Autodesk Inventor part; units mm, degrees
ref_plane "a10_to_bolt_XY" through (0, 9, 75) normal (0, 1, 0) x (1, 0, 0)
ref_plane "a10_to_bolt_YZ" through (0, 9, 75) normal (1, 0, 0) x (0, 0, -1)
ref_plane "a10_to_bolt_ZX" through (0, 9, 75) normal (0, 0, -1) x (0, 1, 0)
sketch "Sketch_1" plane through (0, 0, 0) normal (1, 0, 0) x (0, 1, 0)
  line L0 (0, 55) -> (0, 0)
  line L1 (0, 0) -> (85, 0)
  line L2 (85, 0) -> (85, 9)
  line L3 (85, 9) -> (33, 9)
  line L4 (33, 9) -> (9, 33)
  line L5 (9, 33) -> (9, 55)
  line L6 (9, 55) -> (0, 55)
  arc A0 (8.7071, 30.4645) -> (7, 29.7574) centre (8, 29.7574) ccw
  line L7 (7, 29.7574) -> (7, 12)
  line L8 (7, 12) -> (8.9, 12)
  arc A1 (12.5383, 15.0529) -> (8.9, 12) centre (12, 12) ccw
  line L9 (12.5383, 15.0529) -> (12.3647, 14.0681)
  arc A2 (12.3647, 14.0681) -> (14.0681, 12.3647) centre (12.5843, 12.5843) ccw
  line L10 (14.0681, 12.3647) -> (15.0529, 12.5383)
  arc A3 (12, 8.9) -> (15.0529, 12.5383) centre (12, 12) ccw
  line L11 (12, 8.9) -> (12, 7)
  line L12 (12, 7) -> (29.7574, 7)
  arc A4 (29.7574, 7) -> (30.4645, 8.7071) centre (29.7574, 8) ccw
  line L13 (30.4645, 8.7071) -> (8.7071, 30.4645)
extrude "Extrusion1" add sketch "Sketch_1" along normal mid plane 20
sketch "Sketch_10" plane through (0, 12, 0) normal (0, 1, 0) x (1, 0, 0)
  line L0 (-10, -12) -> (10, -12)
  line L1 (10, -12) -> (10, -14.5)
  line L2 (10, -14.5) -> (9.567, -14.067)
  line L3 (9.567, -14.067) -> (-9.567, -14.067)
  line L4 (-9.567, -14.067) -> (-10, -14.5)
  line L5 (-10, -14.5) -> (-10, -12)
  line L6 (-10, -12) -> (10, -12)
revolve "Revolution1" cut sketch "Sketch_10" angle 360 about axis through (-10, 12, 12) along (-1, 0, 0)
thread "Thread1"
sketch "Sketch3" plane through (10, 0, 0) normal (0, 0, -1) x (-1, 0, 0)
  point P0 (10, 45)
hole "Hole1" at (0, 45, 0) direction (0, 0, 1) diameter 7 depth 9
sketch "Sketch4" plane through (-10, 0, 55) normal (0, -1, 0) x (1, 0, 0)
  point P0 (10, -10)
hole "Hole2" at (0, 0, 45) direction (0, 1, 0) diameter 7 depth 9
sketch "Sketch5" plane through (10, 0, 0) normal (0, 0, -1) x (-1, 0, 0)
  point P0 (10, 75)
hole "Hole3" at (0, 75, 0) direction (0, 0, 1) diameter 7 depth 9
ref_plane "a10_to_bolt_XY" through (0, 9, 75) normal (0, 1, 0) x (1, 0, 0)
ref_plane "a10_to_bolt_YZ" through (0, 9, 75) normal (1, 0, 0) x (0, 0, -1)
ref_plane "a10_to_bolt_ZX" through (0, 9, 75) normal (0, 0, -1) x (0, 1, 0)
ref_plane "a11_to_bolt_XY" through (0, 75, 9) normal (0, 0, 1) x (1, 0, 0)
ref_plane "a11_to_bolt_YZ" through (0, 75, 9) normal (1, 0, 0) x (0, 1, 0)
ref_plane "a11_to_bolt_ZX" through (0, 75, 9) normal (0, 1, 0) x (0, 0, 1)
ref_plane "a13_to_bolt_XY" through (20, 75, 9) normal (0, 0, 1) x (1, 0, 0)
ref_plane "a13_to_bolt_YZ" through (20, 75, 9) normal (1, 0, 0) x (0, 1, 0)
ref_plane "a13_to_bolt_ZX" through (20, 75, 9) normal (0, 1, 0) x (0, 0, 1)
ref_plane "a14_to_bolt_XY" through (-20, 75, 9) normal (0, 0, 1) x (1, 0, 0)
ref_plane "a14_to_bolt_YZ" through (-20, 75, 9) normal (1, 0, 0) x (0, 1, 0)
ref_plane "a14_to_bolt_ZX" through (-20, 75, 9) normal (0, 1, 0) x (0, 0, 1)
ref_plane "a15_to_bolt_XY" through (20, 45, 9) normal (0, 0, 1) x (1, 0, 0)
ref_plane "a15_to_bolt_YZ" through (20, 45, 9) normal (1, 0, 0) x (0, 1, 0)
ref_plane "a15_to_bolt_ZX" through (20, 45, 9) normal (0, 1, 0) x (0, 0, 1)
ref_plane "a16_to_bolt_XY" through (-20, 45, 9) normal (0, 0, 1) x (1, 0, 0)
ref_plane "a16_to_bolt_YZ" through (-20, 45, 9) normal (1, 0, 0) x (0, 1, 0)
ref_plane "a16_to_bolt_ZX" through (-20, 45, 9) normal (0, 1, 0) x (0, 0, 1)
ref_plane "a17_to_bolt_XY" through (20, 9, 75) normal (0, 1, 0) x (1, 0, 0)
ref_plane "a17_to_bolt_YZ" through (20, 9, 75) normal (1, 0, 0) x (0, 0, -1)
ref_plane "a17_to_bolt_ZX" through (20, 9, 75) normal (0, 0, -1) x (0, 1, 0)
ref_plane "a18_XY" through (-20, 9, 75) normal (0, 1, 0) x (1, 0, 0)
ref_plane "a18_YZ" through (-20, 9, 75) normal (1, 0, 0) x (0, 0, -1)
ref_plane "a18_ZX" through (-20, 9, 75) normal (0, 0, -1) x (0, 1, 0)
ref_plane "a19_to_bolt_XY" through (20, 9, 45) normal (0, 1, 0) x (1, 0, 0)
ref_plane "a19_to_bolt_YZ" through (20, 9, 45) normal (1, 0, 0) x (0, 0, -1)
ref_plane "a19_to_bolt_ZX" through (20, 9, 45) normal (0, 0, -1) x (0, 1, 0)
ref_plane "a1_to_bolt_XY" through (0, 45, 9) normal (0, 0, 1) x (1, 0, 0)
ref_plane "a1_to_bolt_YZ" through (0, 45, 9) normal (1, 0, 0) x (0, 1, 0)
ref_plane "a1_to_bolt_ZX" through (0, 45, 9) normal (0, 1, 0) x (0, 0, 1)
ref_plane "a20_to_bolt_XY" through (-20, 9, 45) normal (0, 1, 0) x (1, 0, 0)
ref_plane "a20_to_bolt_YZ" through (-20, 9, 45) normal (1, 0, 0) x (0, 0, -1)
ref_plane "a20_to_bolt_ZX" through (-20, 9, 45) normal (0, 0, -1) x (0, 1, 0)
ref_plane "a2_to_bolt_XY" through (0, 9, 45) normal (0, 1, 0) x (1, 0, 0)
ref_plane "a2_to_bolt_YZ" through (0, 9, 45) normal (1, 0, 0) x (0, 0, -1)
ref_plane "a2_to_bolt_ZX" through (0, 9, 45) normal (0, 0, -1) x (0, 1, 0)
ref_plane "a3_to_bolt_XY" through (0, 75, 9) normal (0, 0, 1) x (1, 0, 0)
ref_plane "a3_to_bolt_YZ" through (0, 75, 9) normal (1, 0, 0) x (0, 1, 0)
ref_plane "a3_to_bolt_ZX" through (0, 75, 9) normal (0, 1, 0) x (0, 0, 1)
ref_plane "a4_to_bolt_XY" through (0, 75, 9) normal (0, 0, 1) x (1, 0, 0)
ref_plane "a4_to_bolt_YZ" through (0, 75, 9) normal (1, 0, 0) x (0, 1, 0)
ref_plane "a4_to_bolt_ZX" through (0, 75, 9) normal (0, 1, 0) x (0, 0, 1)
ref_plane "a5_to_bolt_XY" through (0, 9, 75) normal (0, 1, 0) x (1, 0, 0)
ref_plane "a5_to_bolt_YZ" through (0, 9, 75) normal (1, 0, 0) x (0, 0, -1)
ref_plane "a5_to_bolt_ZX" through (0, 9, 75) normal (0, 0, -1) x (0, 1, 0)
ref_plane "a6_to_bolt_XY" through (0, 9, 75) normal (0, 1, 0) x (1, 0, 0)
ref_plane "a6_to_bolt_YZ" through (0, 9, 75) normal (1, 0, 0) x (0, 0, -1)
ref_plane "a6_to_bolt_ZX" through (0, 9, 75) normal (0, 0, -1) x (0, 1, 0)
ref_plane "a7_to_bolt_XY" through (0, 75, 9) normal (0, 0, 1) x (1, 0, 0)
ref_plane "a7_to_bolt_YZ" through (0, 75, 9) normal (1, 0, 0) x (0, 1, 0)
ref_plane "a7_to_bolt_ZX" through (0, 75, 9) normal (0, 1, 0) x (0, 0, 1)
ref_plane "a8_to_bolt_XY" through (0, 75, 9) normal (0, 0, 1) x (1, 0, 0)
ref_plane "a8_to_bolt_YZ" through (0, 75, 9) normal (1, 0, 0) x (0, 1, 0)
ref_plane "a8_to_bolt_ZX" through (0, 75, 9) normal (0, 1, 0) x (0, 0, 1)
ref_plane "a9_to_bolt_XY" through (0, 9, 75) normal (0, 1, 0) x (1, 0, 0)
ref_plane "a9_to_bolt_YZ" through (0, 9, 75) normal (1, 0, 0) x (0, 0, -1)
ref_plane "a9_to_bolt_ZX" through (0, 9, 75) normal (0, 0, -1) x (0, 1, 0)
ref_plane "bracket_to_dummy_XY" through (0, 0, 0) normal (0, 1, 0) x (1, 0, 0)
ref_plane "bracket_to_dummy_YZ" through (0, 0, 0) normal (1, 0, 0) x (0, 0, -1)
ref_plane "bracket_to_dummy_ZX" through (0, 0, 0) normal (0, 0, -1) x (0, 1, 0)
ref_plane "h12_to_bolt_XY" through (0, 9, 75) normal (0, 1, 0) x (1, 0, 0)
ref_plane "h12_to_bolt_YZ" through (0, 9, 75) normal (1, 0, 0) x (0, 0, -1)
ref_plane "h12_to_bolt_ZX" through (0, 9, 75) normal (0, 0, -1) x (0, 1, 0)
properties part number "HBLTF6-C_"
Source: CAD feature listing. Evaluate the final solid. Frame: model axes, mm. A direction names the side the tool comes from. Round coordinates to 2 decimals unless told otherwise and drop trailing zeros. Loops run counter-clockwise (first coordinate to the right, second up) from the corner with the lowest first, then second, coordinate; pieces in that order, holes last. Notation, with made-up numbers: M 84.5,25 L 127.5,25 A20 ccw 127.5,61 Z; hole C -29,22.25 d5. An arc over 180 degrees is marked long. Use a Markdown table: item, result. Add a question column.
1. Section query B-B on z = 45. Return the cut outline in (x, y), then the cut area to 3 significant figures.
2. Section query A-A on x = 0. Give the number of separate pieces and of enclosed holes in the cut face, then the cut area to 3 significant figures.
3. Contact query for flat-ended pins moving along their axis: P1, Ø8, axis at x = -1, y = 31, coming from the +Z side; P2, Ø3, axis at x = -4.5, y = 22.5, coming from the +Z side; P3, Ø6, axis at x = -3.5, z = 42.5, coming from the +Y side. Output: stop coordinate, or through.
4. Section query D-D on x = 8.5. Return the cut outline in (y, z), then the cut area to 3 significant figures.
5. Mould query, pull axis X, two halves, no side actions, for faces 1 (the flat face through (0, 85, 4)), 2 (the cylindrical face through (1.341, 78.233, 4.563)), 3 (the conical face through (-9.69, 10.507, 10.397)). Classes: pulls with the +X half, pulls with the -X half, needs draft (parallel to the pull), parting line crosses it, or undercut.
6. Reachability of faces 4 (the flat face through (0, 7, 21)), 5 (the conical face through (9.69, 10.397, 10.507)), 6 (the flat face through (0, 9, 41)) from +Z, -Z, +X, -X, +Y, -Y: full face, straight path, thin tool, end or side. Return the list, or none.
7. Line query: line 1 (Y direction, x = 0, z = 4.25); line 2 (X direction, y = 75, z = 2.5); line 3 (Y direction, x = -7.5, z = 11). Output: solid intervals per line, ascending.
Reported:
| question | item | result |
|---|---|---|
| 1 | outline | M -10,0 L -3.5,0 L -3.5,9 L -10,9 Z; M 3.5,0 L 10,0 L 10,9 L 3.5,9 Z |
| 1 | area | 117 mm² |
| 2 | separate pieces | 4 |
| 2 | enclosed holes | 1 |
| 2 | area | 995 mm² |
| 3 | P1 | stops at z = 15 |
| 3 | P2 | stops at z = 21 |
| 3 | P3 | stops at y = 9 |
| 4 | outline | M 0,0 L 85,0 L 85,9 L 33,9 L 9,33 L 9,55 L 0,55 Z; hole M 7,12 L 8.9,12 A3.1 cw 12.54,15.05 L 12.36,14.07 A1.5 ccw 12.27,14.05 A2.07 ccw long 14.05,12.27 A1.5 ccw 14.07,12.36 L 15.05,12.54 A3.1 cw 12,8.9 L 12,7 L 29.76,7 A1 ccw 30.46,8.71 L 8.71,30.46 A1 ccw 7,29.76 Z |
| 4 | area | 1,180 mm² |
| 5 | face 1 | needs draft |
| 5 | face 2 | undercut |
| 5 | face 3 | pulls with the -X half |
| 6 | face 4 | +X, -X |
| 6 | face 5 | +X |
| 6 | face 6 | +Z, +X, -X, +Y |
| 7 | line 1 | y = 0 to 41.5, 48.5 to 71.5, 78.5 to 85 |
| 7 | line 2 | x = -10 to -3.5, 3.5 to 10 |
| 7 | line 3 | y = 0 to 10.19, 13.81 to 14.93, 28.17 to 31 |
